Verification items for the finished model (mm, model axes). Face numbers are marked on the shaded views. A direction names the side the tool comes from. Coordinates: 2 decimals unless noted, no trailing zeros. Loops run counter-clockwise (first coordinate to the right, second up) from the corner with the lowest first, then second, coordinate; pieces in that order, holes last. Notation, with made-up numbers: (37, 18.25) -> (75, 18.25) arc R25 ccw to (75, 39.25) -> close; hole circle Ø2 at (69, 0). An arc over 180 degrees is marked (long way). Answer as a JSON object with one key per item and string values. Group by question number.
Q1. Cross-section at A-A on z = -23.5. Record the boundary of the cut face in (x, y).
Q2. Scan lines: L1, parallel to X at y = -0.5, z = -23.5; L2, parallel to X at y = -2.3, z = 3.5; L3, parallel to Z at x = -3, y = -1. Record each from-to range of solid material in increasing order.
Q3. Release check for a two-part mould opening along X. For the marked faces 4, 5 and 6 record: released by +X, released by -X, zero draft, split by the parting line, or undercut.
Q4. Set-up check for the marked faces 1, 2 and 3: record each of +Z, -Z, +X, -X, +Y, -Y from which the full face is reachable in a straight line by a thin tool's end or side.
Q5. Cross-section at B-B on x = -3. Record the boundary of the cut face in (y, z).
Q6. Cross-section at C-C on y = 34.5. Record the boundary of the cut face in (x, z).
Q7. Gauge pin test, flat ends, axial feed: pin 1 Ø6 at (x, y) = (-1, 37) entering from +Z; pin 2 Ø1.7 at (x, y) = (6, 40) entering from -Z; pin 3 Ø16 at (y, z) = (25.5, -10) entering from +X; pin 4 Ø2.5 at (x, z) = (-3, 3.5) entering from +Y. Record the tip position at first contact, or that the pin passes through.
Autodesk Inventor part; units mm, degrees
ref_plane "YZ Plane" through (0, 0, 0) normal (1, 0, 0) x (0, 1, 0)
ref_plane "XZ Plane" through (0, 0, 0) normal (0, 1, 0) x (-1, 0, 0)
ref_plane "XY Plane" through (0, 0, 0) normal (0, 0, 1) x (1, 0, 0)
sketch "底面" plane through (0, 0, 0) normal (0, 1, 0) x (-1, 0, 0)
  line L0 (0, 0) -> (-16, 0)
  line L1 (-16, 0) -> (-16, -20)
  line L2 (-16, -20) -> (0, -20)
  line L3 (0, -20) -> (0, 0)
  dimension "d0" = 16
  dimension "d1" = 20
extrude "本体" add sketch "底面" along normal blind 50
sketch "ねじ穴スケッチ" plane through (0, 0, 0) normal (0, 0, 1) x (1, 0, 0)
  circle A0 centre (6, 40) radius 1.45
  line L0 (0, 50) -> (16, 50)
  line L1 (16, 0) -> (16, 50)
  point P0 (0, 0)
  dimension "d6" = 10
  dimension "d9" = 2.9
  dimension "d17" = 10
extrude "ねじ穴" cut sketch "ねじ穴スケッチ" against normal blind 12
sketch "接合部スケッチ" plane through (0, 0, 0) normal (0, 0, 1) x (1, 0, 0)
  circle A0 centre (6, 40) radius 1.45
  circle A1 centre (6, 40) radius 4
  point P0 (0, 0)
  dimension "d10" = 8
extrude "接合部" cut sketch "接合部スケッチ" against normal blind 8
sketch "スケッチ4" plane through (6, 40, -8) normal (0, 0, 1) x (1, 0, 0)
  line L0 (2.7, 0) -> (1.35, -2.3383)
  line L1 (1.35, -2.3383) -> (-1.35, -2.3383)
  line L2 (-1.35, -2.3383) -> (-2.7, 0)
  line L3 (-2.7, 0) -> (-1.35, 2.3383)
  line L4 (-1.35, 2.3383) -> (1.35, 2.3383)
  line L5 (1.35, 2.3383) -> (2.7, 0)
  circle A0 centre (0, 0) radius 1.45
  point P0 (-6, -40)
  point P1 (0, 2.3383)
  dimension "d13" = 2.7
  dimension "d14" = 5.4
extrude "ナット穴" cut sketch "スケッチ4" against normal blind 2.4
fillet "フィレット1" radius 8 2 edges at (16, 50, -10) (0, 50, -10)
sketch "スケッチ5" plane through (0, 0, 0) normal (0, -1, 0) x (1, 0, 0)
  line L0 (23, 7.5) -> (-7, 7.5)
  line L1 (-7, 7.5) -> (-7, -27.5)
  line L2 (-7, -27.5) -> (23, -27.5)
  line L3 (23, -27.5) -> (23, 7.5)
  line L4 (0, 0) -> (16, 0)
  line L5 (16, 0) -> (16, -20)
  line L6 (0, -20) -> (0, 0)
  line L7 (16, -20) -> (0, -20)
  line L8 (0, 0) -> (16, 0)
  line L9 (16, 0) -> (16, -20)
  point P0 (8, 7.5)
  point P1 (8, 0)
  point P2 (23, -10)
  point P3 (16, -10)
  dimension "d42" = 30
  dimension "d43" = 35
extrude "足場" add sketch "スケッチ5" along normal blind 3 contours L3 L2 L1 L0 | L4 L5 L7 L6
sketch "スケッチ6" plane through (8, 42, 0) normal (0, 0, 1) x (1, 0, 0)
  circle A0 centre (6, -7.5) radius 1
  line L0 (15, -42) -> (-15, -42)
  line L1 (-8, -42) -> (-8, 0)
  line L2 (8, -42) -> (8, 0)
  dimension "d25" = 2
  dimension "d26" = 34.5
  dimension "d31" = 2
extrude "ストッパー" add sketch "スケッチ6" along normal blind 2.5
sketch "スケッチ7" plane through (0, -3, 0) normal (0, -1, 0) x (1, 0, 0)
  circle A0 centre (-3, 3.5) radius 1.5
  circle A1 centre (19, 3.5) radius 1.5
  circle A2 centre (19, -23.5) radius 1.5
  circle A3 centre (-3, -23.5) radius 1.5
  line L0 (-7, 7.5) -> (-7, -27.5)
  line L1 (23, 7.5) -> (-7, 7.5)
  line L2 (23, -27.5) -> (23, 7.5)
  line L3 (-7, -27.5) -> (23, -27.5)
  dimension "d32" = 3
  dimension "d33" = 3
  dimension "d34" = 3
  dimension "d35" = 3
  dimension "d36" = 4
  dimension "d37" = 4
  dimension "d38" = 4
  dimension "d39" = 4
extrude "押し出し7" cut sketch "スケッチ7" against normal through all contours A0 | A1 | A2 | A3
sketch "スケッチ8" plane through (0, 0, 0) normal (0, 1, 0) x (1, 0, 0)
  circle A0 centre (-3, 23.5) radius 1.5
  circle A1 centre (-3, 23.5) radius 2.85
  circle A2 centre (19, 23.5) radius 2.85
  circle A3 centre (-3, -3.5) radius 2.85
  circle A4 centre (19, -3.5) radius 2.85
  circle A5 centre (19, 23.5) radius 1.5
  circle A6 centre (19, -3.5) radius 1.5
  circle A7 centre (-3, -3.5) radius 1.5
  point P0 (0, 0)
  dimension "d44" = 5.7
  dimension "d45" = 5.7
  dimension "d46" = 5.7
  dimension "d47" = 5.7
extrude "ネジ溝" cut sketch "スケッチ8" against normal blind 1.5
fillet "フィレット2" radius 0.2 4 edges at (8, -3, 7.5) (23, -3, -10) (8, -3, -27.5) (-7, -3, -10)
equation "\"d17\" = d6"
equation "\"d37\" = d36"
equation "\"d38\" = d36"
equation "\"d39\" = d36"
equation "\"d45\" = d44"
equation "\"d46\" = d44"
equation "\"d47\" = d44"
properties part number "body-2_3D プリント"
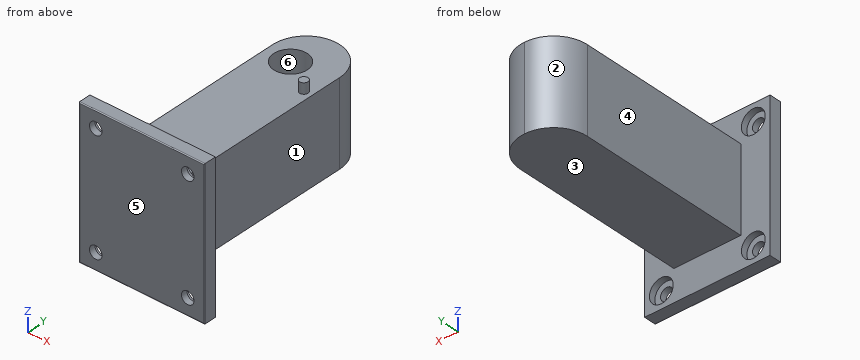
Computed values:
{
 "1": {"outline": "(-7, -2.8) arc R0.2 ccw to (-6.8, -3) -> (-4.5, -3) -> (-4.5, -1.5) -> (-5.85, -1.5) -> (-5.85, 0) -> (-7, 0) -> close; (-1.5, -3) -> (17.5, -3) -> (17.5, -1.5) -> (16.15, -1.5) -> (16.15, 0) -> (-0.15, 0) -> (-0.15, -1.5) -> (-1.5, -1.5) -> close; (20.5, -3) -> (22.8, -3) arc R0.2 ccw to (23, -2.8) -> (23, 0) -> (21.85, 0) -> (21.85, -1.5) -> (20.5, -1.5) -> close"},
 "2": {"L1": "x = -7 to -5.85, -0.15 to 16.15, 21.85 to 23", "L2": "x = -7 to -4.5, -1.5 to 17.5, 20.5 to 23", "L3": "z = -27.5 to -26.35, -20.65 to 0.65, 6.35 to 7.5"},
 "3": {"face 4": "released by -X", "face 5": "zero draft", "face 6": "undercut"},
 "4": {"face 1": "+Z, -Z, +X, +Y", "face 2": "+Z, -Z, -X, +Y", "face 3": "-Z, +X, -X, +Y"},
 "5": {"outline": "(-3, -27.3) arc R0.2 ccw to (-2.8, -27.5) -> (0, -27.5) -> (0, -26.35) -> (-1.5, -26.35) -> (-1.5, -25) -> (-3, -25) -> close; (-3, -22) -> (-1.5, -22) -> (-1.5, -20.65) -> (0, -20.65) -> (0, 0.65) -> (-1.5, 0.65) -> (-1.5, 2) -> (-3, 2) -> close; (-3, 5) -> (-1.5, 5) -> (-1.5, 6.35) -> (0, 6.35) -> (0, 7.5) -> (-2.8, 7.5) arc R0.2 ccw to (-3, 7.3) -> close"},
 "6": {"outline": "(0, -20) -> (16, -20) -> (16, 0) -> (15, 0) -> (15, 2.5) -> (13, 2.5) -> (13, 0) -> (0, 0) -> close"},
 "7": {"pin 1": "stops at z = 0", "pin 2": "stops at z = -20", "pin 3": "stops at x = 16", "pin 4": "passes through"}
}
